from build123d import *

# Parameters (mm, degrees)
SKETCH1_W            = 13.25
SKETCH1_H            = 7.5
SKETCH1_W_2          = 2
SKETCH1_W_3          = 2.24
SKETCH1_W_4          = 3.26
SKETCH1_W_5          = 8.01
SKETCH1_H_2          = 3.25
SKETCH1_H_3          = 2
SKETCH1_R            = 1.25
BOSS_EXTRUDE1_DEPTH  = 1.5
M2_CLEARANCE_HOLE1_D = 2.4
FILLET1_R            = 1


with BuildPart() as part:
    # Sketch1 → Boss-Extrude1 (new body)
    # profile 1 of 22: a face of its own
    with BuildSketch(Plane(origin=(0, 0, 0), x_dir=(1, 0, 0), z_dir=(0, 1, 0))):
        with Locations((-9.375, 0)):
            Rectangle(SKETCH1_W, SKETCH1_H)
    # profile 2 of 22: a face of its own
    with BuildSketch(Plane(origin=(0, 0, 0), x_dir=(1, 0, 0), z_dir=(0, 1, 0))):
        with Locations((-17, 0)):
            Rectangle(SKETCH1_W_2, SKETCH1_H)
    # profile 3 of 22: a face of its own
    with BuildSketch(Plane(origin=(0, 0, 0), x_dir=(1, 0, 0), z_dir=(0, 1, 0))):
        with Locations((-1.63, 0)):
            Rectangle(SKETCH1_W_3, SKETCH1_H)
    # profile 4 of 22: a face of its own
    with BuildSketch(Plane(origin=(0, 0, 0), x_dir=(1, 0, 0), z_dir=(0, 1, 0))):
        with Locations((1.12, 0)):
            Rectangle(SKETCH1_W_4, SKETCH1_H)
    # profile 5 of 22: a face of its own
    with BuildSketch(Plane(origin=(0, 0, 0), x_dir=(1, 0, 0), z_dir=(0, 1, 0))):
        with Locations((3.87, 0)):
            Rectangle(SKETCH1_W_3, SKETCH1_H)
    # profile 6 of 22: a face of its own
    with BuildSketch(Plane(origin=(0, 0, 0), x_dir=(1, 0, 0), z_dir=(0, 1, 0))):
        with Locations((8.995, 0)):
            Rectangle(SKETCH1_W_5, SKETCH1_H)
    # profile 7 of 22: a face of its own
    with BuildSketch(Plane(origin=(0, 0, 0), x_dir=(1, 0, 0), z_dir=(0, 1, 0))):
        with Locations((14, 0)):
            Rectangle(SKETCH1_W_2, SKETCH1_H)
    # profile 8 of 22: a face of its own
    with BuildSketch(Plane(origin=(0, 0, 0), x_dir=(1, 0, 0), z_dir=(0, 1, 0))):
        with Locations((16, 0)):
            Rectangle(SKETCH1_W_2, SKETCH1_H)
    # profile 9 of 22: a face of its own
    with BuildSketch(Plane(origin=(0, 0, 0), x_dir=(1, 0, 0), z_dir=(0, 1, 0))):
        with Locations((3.87, 5.375)):
            Rectangle(SKETCH1_W_3, SKETCH1_H_2)
    # profile 10 of 22: a face of its own
    with BuildSketch(Plane(origin=(0, 0, 0), x_dir=(1, 0, 0), z_dir=(0, 1, 0))):
        with Locations((3.87, -5.375)):
            Rectangle(SKETCH1_W_3, SKETCH1_H_2)
    # profile 11 of 22: a face of its own
    with BuildSketch(Plane(origin=(0, 0, 0), x_dir=(1, 0, 0), z_dir=(0, 1, 0))):
        with Locations((3.87, -8)):
            Rectangle(SKETCH1_W_3, SKETCH1_H_3)
    # profile 12 of 22: a face of its own
    with BuildSketch(Plane(origin=(0, 0, 0), x_dir=(1, 0, 0), z_dir=(0, 1, 0))):
        with Locations((1.12, -8)):
            Rectangle(SKETCH1_W_4, SKETCH1_H_3)
    # profile 13 of 22: a face of its own
    with BuildSketch(Plane(origin=(0, 0, 0), x_dir=(1, 0, 0), z_dir=(0, 1, 0))):
        with Locations((1.12, -5.375)):
            Rectangle(SKETCH1_W_4, SKETCH1_H_2)
    # profile 14 of 22: a face of its own
    with BuildSketch(Plane(origin=(0, 0, 0), x_dir=(1, 0, 0), z_dir=(0, 1, 0))):
        with Locations((1.12, 5.375)):
            Rectangle(SKETCH1_W_4, SKETCH1_H_2)
    # profile 15 of 22: a face of its own
    with BuildSketch(Plane(origin=(0, 0, 0), x_dir=(1, 0, 0), z_dir=(0, 1, 0))):
        with Locations((1.12, 8)):
            Rectangle(SKETCH1_W_4, SKETCH1_H_3)
    # profile 16 of 22: a face of its own
    with BuildSketch(Plane(origin=(0, 0, 0), x_dir=(1, 0, 0), z_dir=(0, 1, 0))):
        with Locations((3.87, 8)):
            Rectangle(SKETCH1_W_3, SKETCH1_H_3)
    # profile 17 of 22: a face of its own
    with BuildSketch(Plane(origin=(0, 0, 0), x_dir=(1, 0, 0), z_dir=(0, 1, 0))):
        with BuildLine():
            Line((2.75, 9.125), (2.75, 11.2072))
            ThreePointArc((2.75, 11.2072), (0, 13.9572), (-2.75, 11.2072))
            Line((-2.75, 11.2072), (-2.75, 9.125))
            Line((-2.75, 9.125), (2.75, 9.125))
        make_face()
        with Locations((0, 11.2072)):
            Circle(SKETCH1_R, mode=Mode.SUBTRACT)
    # profile 18 of 22: a face of its own
    with BuildSketch(Plane(origin=(0, 0, 0), x_dir=(1, 0, 0), z_dir=(0, 1, 0))):
        with BuildLine():
            Line((2.75, -11.2072), (2.75, -9.125))
            Line((2.75, -9.125), (-2.75, -9.125))
            Line((-2.75, -9.125), (-2.75, -11.2072))
            ThreePointArc((-2.75, -11.2072), (0, -13.9572), (2.75, -11.2072))
        make_face()
        with Locations((0, -11.2072)):
            Circle(SKETCH1_R, mode=Mode.SUBTRACT)
    # profile 19 of 22: a face of its own
    with BuildSketch(Plane(origin=(0, 0, 0), x_dir=(1, 0, 0), z_dir=(0, 1, 0))):
        Polygon((2.75, 9), (2.75, 9.125), (-2.75, 9.125), (-2.75, 9), (-0.51, 9), align=None)
    # profile 20 of 22: a face of its own
    with BuildSketch(Plane(origin=(0, 0, 0), x_dir=(1, 0, 0), z_dir=(0, 1, 0))):
        with Locations((0, 11.2072)):
            Circle(SKETCH1_R)
    # profile 21 of 22: a face of its own
    with BuildSketch(Plane(origin=(0, 0, 0), x_dir=(1, 0, 0), z_dir=(0, 1, 0))):
        with Locations((0, -11.2072)):
            Circle(SKETCH1_R)
    # profile 22 of 22: a face of its own
    with BuildSketch(Plane(origin=(0, 0, 0), x_dir=(1, 0, 0), z_dir=(0, 1, 0))):
        Polygon((2.75, -9.125), (2.75, -9), (-0.51, -9), (-2.75, -9), (-2.75, -9.125), align=None)
    extrude(amount=BOSS_EXTRUDE1_DEPTH)

    # M2 Clearance Hole1 (through all)
    with Locations(Plane(origin=(0, 0, -11.2072), x_dir=(0, 0, -1), z_dir=(0, -1, 0))):
        with Locations((0, 0), (-22.4144, 0)):
            Hole(M2_CLEARANCE_HOLE1_D / 2)

    # Fillet1
    fillet1_edges = [part.edges().sort_by_distance(p)[0] for p in [
        (-0.51, 0.75, 3.75),
        (-18, 0.75, 3.75),
        (-18, 0.75, -3.75),
        (-0.51, 0.75, -3.75),
        (-0.51, 0.75, -9),
        (-2.75, 0.75, -9),
        (2.75, 0.75, -9),
        (4.99, 0.75, -9),
        (4.99, 0.75, -3.75),
        (17, 0.75, -3.75),
        (17, 0.75, 3.75),
        (4.99, 0.75, 3.75),
        (4.99, 0.75, 9),
        (2.75, 0.75, 9),
        (-2.75, 0.75, 9),
        (-0.51, 0.75, 9),
    ]]
    fillet(fillet1_edges, radius=FILLET1_R)


solid = part.part
For this review, take the finished solid that the model builds, in its own axes (mm). A direction names the side the tool comes from. Coordinates: 2 decimals unless noted, no trailing zeros. Order: outer loops, then holes, each group sorted by start corner. A loop starts at its lowest first (then second) coordinate and runs counter-clockwise, first axis right, second up. Notation, with made-up numbers: (6, 52.25) -> (21, 52.25) arc R13 ccw to (21, 74.25) -> close; hole circle Ø4 at (55, -4.5). An arc over 180 degrees is marked (long way). Return JSON: item names as keys, results as strings.
1. For pin 1 Ø0.8 at (y, z) = (0.5, -7) entering from +X; pin 2 Ø1.4 at (x, z) = (0, 11.21) entering from +Y, all flat-tipped, find the tip position at first contact; note any pin that passes through.
Answer block:
{"pin 1": "x = 4.99", "pin 2": "through"}
2. We need section B-B on z = 5.5. Write out the cut boundary in (x, y), and give its area (3 significant figures).
Answer block:
{"outline": "(-0.51, 0) -> (4.99, 0) -> (4.99, 1.5) -> (-0.51, 1.5) -> close", "area": "8.25 mm²"}
3. We need section D-D on x = -7. Write out the cut boundary in (y, z), and give its area (4 significant figures).
Answer block:
{"outline": "(0, -3.75) -> (1.5, -3.75) -> (1.5, 3.75) -> (0, 3.75) -> close", "area": "11.25 mm²"}
4. The part is to be moulded in two halves that separate along X. For faces 5 (the cylindrical face through (0.36, 0.76, 12.35)), 6 (the cylindrical face through (3.051, 0.76, -9.285)), 7 (the cylindrical face through (-0.811, 0.76, -4.035)), say which applies: +X half, -X half, draft (parallel to the pull), parting line (faces both ways), or undercut.
Answer block:
{"face 5": "undercut", "face 6": "+X half", "face 7": "-X half"}
5. For line 1 (Z direction, x = -1.5, y = 0.65); line 2 (X direction, y = 0.65, z = 5); line 3 (Z direction, x = 12.5, y = 1.2), list the stretches that pass through material, from the lowest coordinate up. Write a range as from..to.
Answer block:
{"line 1": "-13.51..-9, -3.75..3.75, 9..13.51", "line 2": "-0.51..4.99", "line 3": "-3.75..3.75"}
6. Machinability: for faces 1 (the flat face through (2.75, 1, 11)), 2 (the flat face through (-2.75, 1, 11)), 3 (the flat face through (11, 1, -3.75)), 4 (the cylindrical face through (-2.465, 0.76, 9.301)), which of the approach directions +Z, -Z, +X, -X, +Y, -Y give a long, thin tool a straight path to every point of the face, cutting with its end or side? Answer none if there is none.
Answer block:
{"face 1": "+Z, +X, +Y, -Y", "face 2": "+Z, -X, +Y, -Y", "face 3": "-Z, +X, +Y, -Y", "face 4": "-X, +Y, -Y"}
7. We need section C-C on y = 0.45. State how many separate pieces and enclosed holes the cut face has, and give its area (3 significant figures).
Answer block:
{"separate pieces": "1", "enclosed holes": "2", "area": "359 mm²"}
8. We need section A-A on x = 0. Write out the cut boundary in (y, z), and give its area (3 significant figures).
Answer block:
{"outline": "(0, -13.96) -> (1.5, -13.96) -> (1.5, -12.41) -> (0, -12.41) -> close; (0, -10.01) -> (1.5, -10.01) -> (1.5, 10.01) -> (0, 10.01) -> close; (0, 12.41) -> (1.5, 12.41) -> (1.5, 13.96) -> (0, 13.96) -> close", "area": "34.7 mm²"}
